Autodesk Inventor part; units mm, degrees
ref_plane "YZ Plane" through (0, 0, 0) normal (1, 0, 0) x (0, 1, 0)
ref_plane "XZ Plane" through (0, 0, 0) normal (0, 1, 0) x (-1, 0, 0)
ref_plane "XY Plane" through (0, 0, 0) normal (0, 0, 1) x (1, 0, 0)
sketch "Skizze1" plane through (0, 0, 0) normal (0, 0, 1) x (1, 0, 0)
  line L0 (-20, 10) -> (20, 10)
  line L1 (20, 10) -> (20, -10)
  line L2 (20, -10) -> (-20, -10)
  line L3 (-20, -10) -> (-20, 10)
  line L4 (-28, 0) -> (28, 0)
  line L5 (0, -14) -> (0, 14)
  circle A0 centre (0, 0) radius 5
  dimension "d0" = 40
  dimension "d1" = 20
  dimension "d2" = 10
extrude "Extrusion1" add sketch "Skizze1" along normal blind 10 contours L0 L5 A0 L4 L3 | L0 L1 L4 A0 L5 | L4 A0 L5 L2 L3 | L1 L2 L5 A0 L4
sketch "Skizze2" plane through (0, 0, 0) normal (0, 0, -1) x (-1, 0, 0)
  circle A0 centre (0, 0) radius 5
  circle A1 centre (0, 0) radius 6
  dimension "d5" = 12
extrude "Extrusion2" cut sketch "Skizze2" against normal blind 8
sketch "Skizze3" plane through (0, 0, 10) normal (0, 0, 1) x (1, 0, 0)
  line L0 (-20, 10) -> (20, 10)
  line L1 (20, -10) -> (-20, -10)
  line L2 (-13, 10) -> (-13, -10)
  line L3 (13, -10) -> (13, 10)
  line L4 (-11.2, 1) -> (-11.2, -1)
  line L5 (-14.8, -1) -> (-14.8, 1)
  line L6 (14.8, 1) -> (14.8, -1)
  line L7 (11.2, -1) -> (11.2, 1)
  line L8 (-28, 0) -> (28, 0)
  line L9 (0, -14) -> (0, 14)
  arc A0 (-11.2, 1) -> (-14.8, 1) centre (-13, 1) ccw
  arc A1 (-14.8, -1) -> (-11.2, -1) centre (-13, -1) ccw
  arc A2 (11.2, -1) -> (14.8, -1) centre (13, -1) ccw
  arc A3 (14.8, 1) -> (11.2, 1) centre (13, 1) ccw
  dimension "d8" = 26
  dimension "d9" = 3.6
  dimension "d11" = 2
extrude "Extrusion3" cut sketch "Skizze3" against normal through all contours A0 L4 L8 L2 | L2 L8 L5 A0 | L8 L4 A1 L2 | L2 A1 L5 L8 | A3 L6 L8 L3 | L3 L8 L7 A3 | L8 L3 A2 L7 | L8 L6 A2 L3
sketch "Skizze4" plane through (0, 0, 10) normal (0, 0, 1) x (1, 0, 0)
  arc A0 (-14.8, -1) -> (-11.2, -1) centre (-13, -1) ccw
  line L0 (-14.8, -1) -> (-14.8, 1)
  arc A1 (-11.2, 1) -> (-14.8, 1) centre (-13, 1) ccw
  line L1 (-11.2, 1) -> (-11.2, -1)
  arc A2 (11.2, -1) -> (14.8, -1) centre (13, -1) ccw
  line L2 (11.2, -1) -> (11.2, 1)
  arc A3 (14.8, 1) -> (11.2, 1) centre (13, 1) ccw
  line L3 (14.8, 1) -> (14.8, -1)
  line L4 (-16.5, 1) -> (-16.5, -1)
  arc A4 (-16.5, -1) -> (-9.5, -1) centre (-13, -1) ccw
  line L5 (-9.5, -1) -> (-9.5, 1)
  arc A5 (-9.5, 1) -> (-16.5, 1) centre (-13, 1) ccw
  line L6 (9.5, 1) -> (9.5, -1)
  arc A6 (9.5, -1) -> (16.5, -1) centre (13, -1) ccw
  line L7 (16.5, -1) -> (16.5, 1)
  arc A7 (16.5, 1) -> (9.5, 1) centre (13, 1) ccw
  dimension "d14" = 7
extrude "Extrusion4" cut sketch "Skizze4" against normal blind 5
properties part number "13_0204_057"
The listing builds one solid part. Answer for the finished solid, in the listing's coordinates (mm). A direction names the side the tool comes from. Coordinates: 2 decimals unless noted, no trailing zeros. Write each loop counter-clockwise with the first axis right and the second up, starting at its lowest first coordinate (ties: lowest second). Pieces come first, ordered by that corner, then holes. Notation, with made-up numbers: (65.25, 2) - (87.25, 2) arc R20 ccw to (87.25, 30) - close; hole circle Ø3 at (-22, 16). An arc over 180 degrees is marked (long way). Return JSON: item names as keys, results as strings.
1. The part is cut by section C-C on y = 0. Determine the outline of the cut face in (x, z).
Final values:
{"outline": "(-20, 0) - (-14.8, 0) - (-14.8, 5) - (-16.5, 5) - (-16.5, 10) - (-20, 10) - close; (-11.2, 0) - (-6, 0) - (-6, 8) - (-5, 8) - (-5, 10) - (-9.5, 10) - (-9.5, 5) - (-11.2, 5) - close; (5, 8) - (6, 8) - (6, 0) - (11.2, 0) - (11.2, 5) - (9.5, 5) - (9.5, 10) - (5, 10) - close; (14.8, 0) - (20, 0) - (20, 10) - (16.5, 10) - (16.5, 5) - (14.8, 5) - close"}
2. The part is cut by section A-A on x = 13. Determine the outline of the cut face in (y, z).
Final values:
{"outline": "(-10, 0) - (-2.8, 0) - (-2.8, 5) - (-4.5, 5) - (-4.5, 10) - (-10, 10) - close; (2.8, 0) - (10, 0) - (10, 10) - (4.5, 10) - (4.5, 5) - (2.8, 5) - close"}
3. The part is cut by section B-B on z = 3.25. Determine the outline of the cut face in (x, y), then the cut area to 3 significant figures.
Final values:
{"outline": "(-20, -10) - (20, -10) - (20, 10) - (-20, 10) - close; hole (-14.8, -1) arc R1.8 ccw to (-11.2, -1) - (-11.2, 1) arc R1.8 ccw to (-14.8, 1) - close; hole circle Ø12 at (0, 0); hole (11.2, -1) arc R1.8 ccw to (14.8, -1) - (14.8, 1) arc R1.8 ccw to (11.2, 1) - close", "area": "652 mm^2"}
4. Which of the six approach directions +Z, -Z, +X, -X, +Y, -Y give full straight-line access (tool end or side, diameter ignored) to faces 4 (the face through (13, -2.8, 2.5)), 5 (the face through (4, 4, 8)), 6 (the face through (9.5, 0, 8))?
Final values:
{"face 4": "+Z, -Z", "face 5": "-Z", "face 6": "+Z"}
5. Consider line 1 along X through (y, z) = (0, 8.55); line 2 along Y through (x, z) = (0, 2.25); line 3 along Y through (x, z) = (0, 9). Determine where each line is inside the solid, lowest interval first.
Final values:
{"line 1": "-20 to -16.5, -9.5 to -5, 5 to 9.5, 16.5 to 20", "line 2": "-10 to -6, 6 to 10", "line 3": "-10 to -5, 5 to 10"}
6. This flat-tipped pin is pushed along its axis until it touches: pin 1 Ø3.5 at (x, y) = (-14, 0) entering from +Z. Where does it stop, or does it pass through?
Final values:
{"pin 1": "z = 5"}
7. The part is cut by section D-D on x = 0. Determine the outline of the cut face in (y, z).
Final values:
{"outline": "(-10, 0) - (-6, 0) - (-6, 8) - (-5, 8) - (-5, 10) - (-10, 10) - close; (5, 8) - (6, 8) - (6, 0) - (10, 0) - (10, 10) - (5, 10) - close"}
8. For a pull along X with two mould halves and no side action, classify faces 1 (the face through (-9.5, 0, 8)), 2 (the face through (-20, 0, 5)), 3 (the face through (0, -10, 5)) as +X half, -X half, draft (parallel to the pull), parting line (faces both ways), or undercut.
Final values:
{"face 1": "undercut", "face 2": "-X half", "face 3": "draft"}
